Can you work these out from the drawing? Everything is in mm from the part's minimum corner. A direction names the side the tool comes from. Give positions to 0.01 mm unless a question says otherwise; leave off trailing zeros. Write each loop counter-clockwise with the first axis right and the second up, starting at its lowest first coordinate (ties: lowest second). Pieces come first, ordered by that corner, then holes. Notation, with made-up numbers: (29, 17) - (85, 17) arc R26 ccw to (85, 55) - close; hole circle Ø7 at (-12.75, 66). An arc over 180 degrees is marked (long way). Use a Markdown table: item, result.
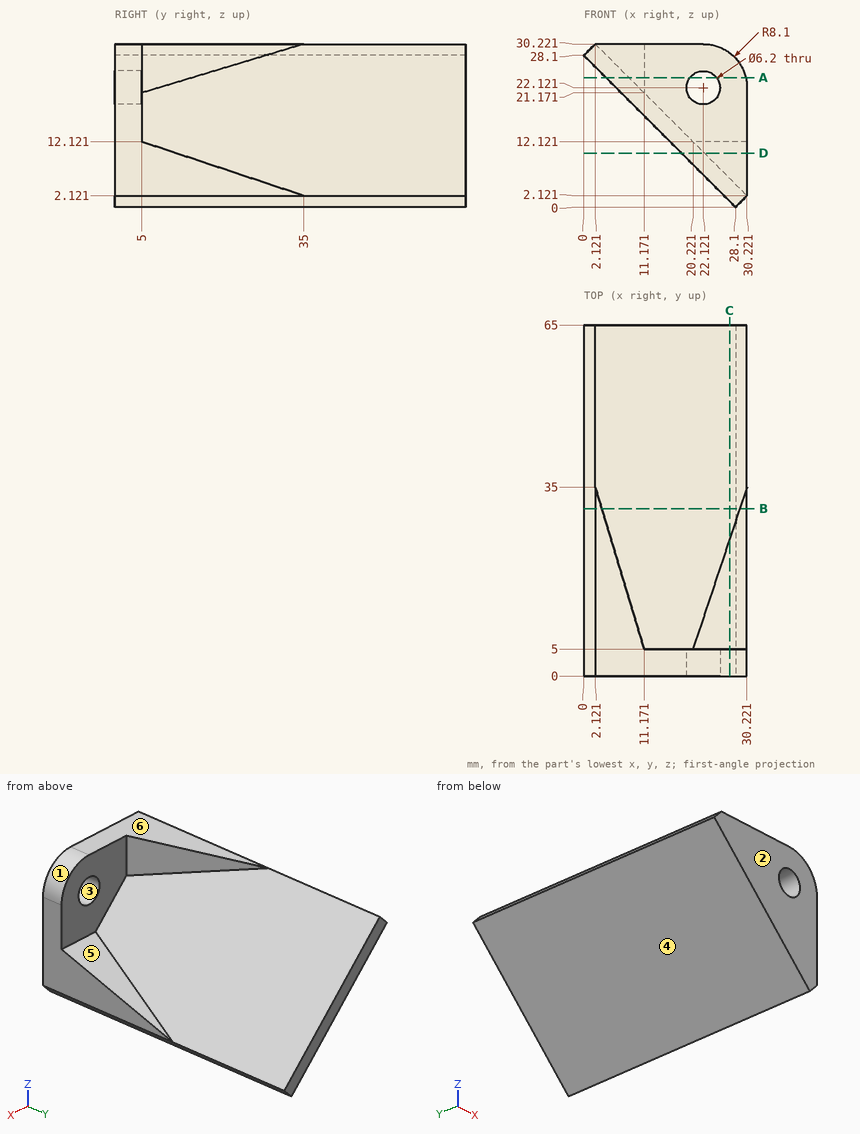
Item 1: If we section it at B-B, the plane y = 31: Write out the boundary of the cut face in (x, z) (1 decimal), plus the area to 3 significant figures.
Values:
| item | result |
|---|---|
| outline | (0, 28.1) - (28.1, 0) - (30.2, 2.1) - (30.2, 3.5) - (28.9, 3.5) - (3.3, 29) - (3.3, 30.2) - (2.1, 30.2) - close |
| area | 121 mm2 |
Item 2: For the marked faces 5 and 6, which set-ups out of +Z, -Z, +X, -X, +Y, -Y let a thin tool reach every point of the face, with its end or its side?
Values:
| item | result |
|---|---|
| face 5 | +Z, +X, +Y |
| face 6 | +Z, +X, -X, +Y, -Y |
Item 3: I need wall thicknesses on line 1 along Y through (x, z) = (23, 17); line 2 along Z through (x, y) = (24, 3.5) (1 decimal); line 3 along X through (y, z) = (57, 13). Which ranges of each line are inside material? Lowest first, please. Write a range as [from, to].
Values:
| item | result |
|---|---|
| line 1 | y = [0, 5] |
| line 2 | z = [4.1, 19.7], [24.6, 30] |
| line 3 | x = [15.1, 19.34] |
Item 4: Thinking about a two-plate mould opening in X: for the marked faces 1, 2, 3 and 4, which applies, +X half, -X half, draft (parallel to the pull), parting line (faces both ways), or undercut?
Values:
| item | result |
|---|---|
| face 1 | +X half |
| face 2 | draft |
| face 3 | undercut |
| face 4 | -X half |
Item 5: If we section it at C-C, the plane x = 27: Write out the boundary of the cut face in (y, z).
Values:
| item | result |
|---|---|
| outline | (0, 1.1) - (65, 1.1) - (65, 5.34) - (25.34, 5.34) - (5, 12.12) - (5, 28.59) - (0, 28.59) - close |
Item 6: If we section it at A-A, the plane z = 24: Write out the boundary of the cut face in (x, y) (1 decimal).
Values:
| item | result |
|---|---|
| outline | (4.1, 0) - (19.7, 0) - (19.7, 5) - (11.2, 5) - (8.3, 14.4) - (8.3, 65) - (4.1, 65) - close; (24.6, 0) - (30, 0) - (30, 5) - (24.6, 5) - close |
Item 7: If we section it at D-D, the plane z = 10: Write out the boundary of the cut face in (x, y).
Values:
| item | result |
|---|---|
| outline | (18.1, 0) - (30.22, 0) - (30.22, 11.36) - (22.34, 11.36) - (22.34, 65) - (18.1, 65) - close |
Item 8: Will these pins go through, and if not, where does the flat tip stop? pin 1 Ø5.5 at (x, z) = (20, 21) entering from +Y; pin 2 Ø6 at (y, z) = (15.5, 26) entering from +X; pin 3 Ø5 at (x, y) = (21.5, 12.5) entering from -Z.
Values:
| item | result |
|---|---|
| pin 1 | stops at y = 5 |
| pin 2 | stops at x = 9.34 |
| pin 3 | stops at z = 4.1 |
